Geometry check sheet. Reference: the model listing, model coordinates, mm. Face numbers are marked on the shaded views. Give positions to 0.01 mm unless a question says otherwise; leave off trailing zeros. Write each question's results on one line, items separated by ' | '. Start each with the question number.
1) Draft check along Z on the marked faces 1, 2 and 3. Enter one of: pulls with the +Z half, pulls with the -Z half, needs draft (parallel to the pull), parting line crosses it, or undercut.
2) Scan lines: line 1 (Z direction, x = -4, y = 16.5); line 2 (X direction, y = 16, z = 9); line 3 (X direction, y = -14, z = 8.5). Record each from-to range of solid material in increasing order. Write a range as from..to.
3) Sectioned sample at A-A on z = 4.5. Count the separate pieces of the cut face and the enclosed holes in it, then the cut area to 3 significant figures.
4) Depth check by flat-ended pin: pin 1 (1 mm diameter, centred on y = 8.5, z = 26.5, fed in from -X); pin 2 (2 mm diameter, centred on y = -13.5, z = 30, fed in from +X); pin 3 (16.5 mm diameter, centred on x = -30.5, y = 1, fed in from +Z). Enter the tip coordinate at first touch or a pass-through.
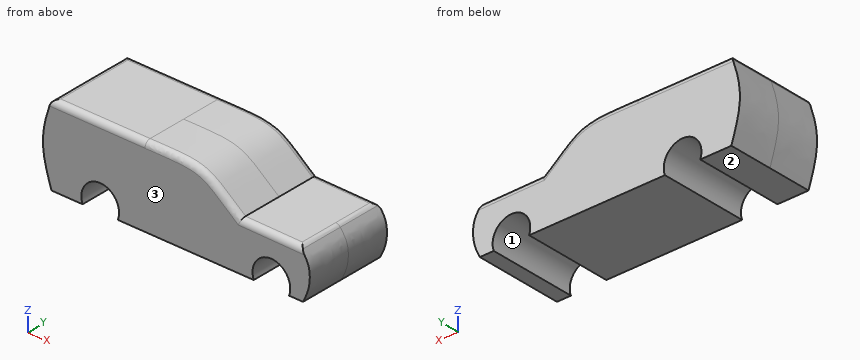
```python
from build123d import *

# Parameters (mm, degrees)
F1_DEPTH = 19.05
F2_R     = 2.54


# Not quite as in the source:
# - a feature of the source that left no trace in its solid (it failed there, or was rolled back) is left out
# - the program builds the solid bodies; features that only make, move or delete a surface that nothing else refers to are left out


with BuildPart() as f1:
    # F0 (on Front) → F1 (new body, symmetric)
    with BuildSketch(Plane.XZ):
        with BuildLine():
            Line((57.1580786184, 0), (63.1808337388, 0))
            add(Edge.make_bspline(
                [(63.1808337388, 0), (64.1070753603, 1.8610503512), (66.0809264552, 5.8270093279), (66.4899415159, 14.6578153912), (63.3565966702, 18.5563140043), (61.8450880558, 20.4369286596)],
                knots=[0, 0, 0, 0, 0.3139594033, 0.669057725, 1, 1, 1, 1], degree=3))
            Line((61.8450880558, 20.4369286596), (36.198740513, 20.7040771047))
            add(Edge.make_bspline(
                [(36.198740513, 20.7040771047), (34.2669116908, 22.189306267), (29.9242250959, 25.5280517601), (20.2820782894, 33.6171914647), (6.7709379775, 34.1670870206), (-1.1152122764, 34.0960294227), (-4.942264819, 34.0615460371)],
                knots=[0, 0, 0, 0, 0.2093274169, 0.4705610335, 0.7430697263, 1, 1, 1, 1], degree=3))
            Line((-4.942264819, 34.0615460371), (-45.2818187647, 34.0615460371))
            add(Edge.make_bspline(
                [(-45.2818187647, 34.0615460371), (-46.4011998646, 30.7970228492), (-48.6607847814, 24.2072498428), (-49.5278252711, 13.2391089732), (-46.7579858308, 4.6027100105), (-45.2818187647, 0)],
                knots=[0, 0, 0, 0, 0.3143769013, 0.6346018389, 1, 1, 1, 1], degree=3))
            Line((-45.2818187647, 0), (-31.8846153722, 0))
            ThreePointArc((-31.8846153722, 0), (-24.2646153722, 10.9564242963), (-16.6446153722, 0))
            Line((-16.6446153722, 0), (41.9180786184, 0))
            ThreePointArc((41.9180786184, 0), (49.5380786184, 10.9564242963), (57.1580786184, 0))
        make_face()
    extrude(amount=F1_DEPTH, both=True)

    # F2
    f2_edges = [f1.edges().sort_by_distance(p)[0] for p in [
        (49.021914, -19.05, 20.570503),
        (49.021914, 19.05, 20.570503),
        (61.845088, 9.525, 20.436929),
        (61.845088, -9.525, 20.436929),
        (17.503149, -19.05, 32.967083),
        (17.503149, 19.05, 32.967083),
        (-45.281819, -9.525, 34.061546),
        (-45.281819, 9.525, 34.061546),
        (-25.112042, 19.05, 34.061546),
        (-25.112042, -19.05, 34.061546),
    ]]
    fillet(f2_edges, radius=F2_R)


solid = f1.part
```
Result:
1) face 1: undercut | face 2: pulls with the -Z half | face 3: needs draft
2) line 1: 0..34.07 | line 2: -47.92..-29.55, -18.98..44.25, 54.83..66.06 | line 3: -47.8..-30.09, -18.44..43.72, 55.36..66.01
3) separate pieces: 3 | enclosed holes: 0 | area: 3,050 mm^2
4) pin 1: x = -47.8 | pin 2: x = 25.57 | pin 3: z = 34.06
